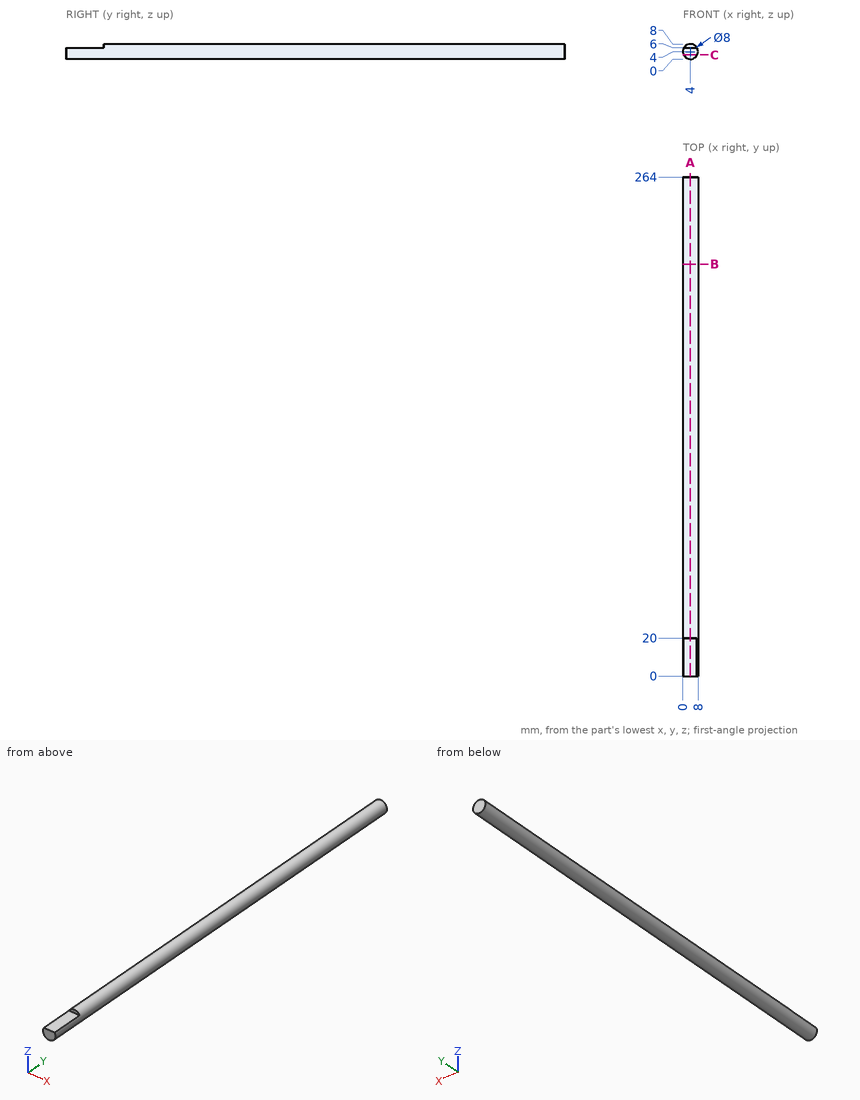
The drawing under review shows one solid part. Ordinate dimensions are in mm from its lowest x, y, z. Give positions to 0.01 mm unless a question says otherwise; leave off trailing zeros. Order: outer loops, then holes, each group sorted by start corner. A loop starts at its lowest first (then second) coordinate and runs counter-clockwise, first axis right, second up. Notation, with made-up numbers: M -12,68 L 43,68 A25 ccw 43,83 Z; hole C -23.75,-27.75 d6. An arc over 180 degrees is marked long. Answer in a Markdown table with one row per item. Add a question column.
1. Add section B-B on y = 218. State the section outline as (x, z) points.
2. To check wall thickness, follow line 1 along Z through (x, y) = (4.5, 187); line 2 along Z through (x, y) = (6, 13). State the ranges of each line that lie inside material, in increasing order.
3. For pin 1 Ø4 at (x, y) = (6.5, 101) entering from -Z; pin 2 Ø2 at (x, y) = (3.5, 10) entering from +Z; pin 3 Ø0.6 at (x, z) = (4.5, 6.5) entering from -Y, all flat-tipped, find the tip position at first contact; note any pin that passes through.
4. Add section A-A on x = 4. State the section outline as (y, z) points, plus the area to 3 significant figures.
5. Add section C-C on z = 2.25. State the section outline as (x, y) points, plus the area to 3 significant figures.
The answers:
| question | item | result |
|---|---|---|
| 1 | outline | C 4,4 d8 |
| 2 | line 1 | 0.03 to 7.97 |
| 2 | line 2 | 0.54 to 6 |
| 3 | pin 1 | z = 0.03 |
| 3 | pin 2 | z = 6 |
| 3 | pin 3 | y = 20 |
| 4 | outline | M 0,0 L 264,0 L 264,8 L 20,8 L 20,6 L 0,6 Z |
| 4 | area | 2,070 mm2 |
| 5 | outline | M 0.4,0 L 7.6,0 L 7.6,264 L 0.4,264 Z |
| 5 | area | 1,900 mm2 |
